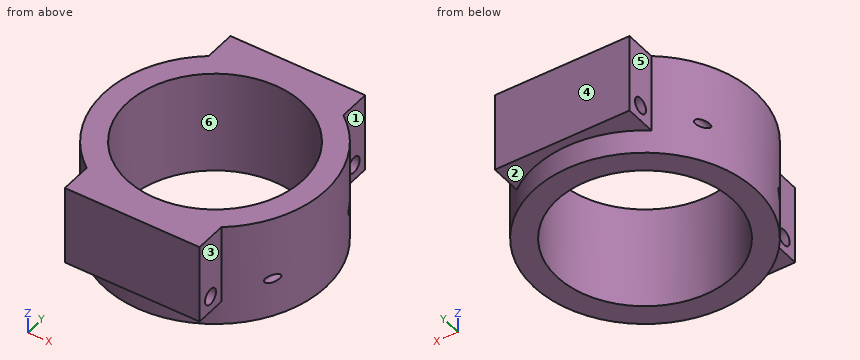
```python
from build123d import *

# Parameters (mm, degrees)
SKETCH_R           = 14
PAD_DEPTH          = 13
SKETCH001_R        = 11.1
POCKET_DEPTH       = 13.001
SKETCH002_W        = 17
SKETCH002_H        = 4
PAD001_DEPTH       = 10
POLARPATTERN_COUNT = 2
SKETCH003_R        = 0.5
POCKET001_DEPTH    = 111.473218
SKETCH004_R        = 1
POCKET002_DEPTH    = 110.373218


with BuildPart() as part:
    # Sketch → Pad (new body)
    with BuildSketch(Plane.XY):
        Circle(SKETCH_R)
    extrude(amount=PAD_DEPTH)

    # Sketch001 → Pocket (cut, through all)
    with BuildSketch(Plane.XY.offset(13)):
        Circle(SKETCH001_R)
    extrude(amount=-POCKET_DEPTH, mode=Mode.SUBTRACT)

    # Sketch002 → Pad001 (new body)
    with BuildSketch(Plane.XY.offset(13)):
        with Locations((0, 13.1)):
            Rectangle(SKETCH002_W, SKETCH002_H)
    pad001 = extrude(amount=-PAD001_DEPTH)

    # PolarPattern: Pad001 ×2 about axis
    polarpattern_axis = Axis((0, 0, 13), (0, 0, 1))
    for i in range(1, POLARPATTERN_COUNT):
        add(pad001.rotate(polarpattern_axis, i * 360 / POLARPATTERN_COUNT))

    # Sketch003 → Pocket001 (cut, through all)
    with BuildSketch(Plane.XZ.offset(10)):
        with Locations((12.1, 5)):
            Circle(SKETCH003_R)
    pocket001 = extrude(amount=-POCKET001_DEPTH, mode=Mode.SUBTRACT)

    # Mirrored: Pocket001 across Sketch003 V_Axis
    add(pocket001.mirror(Plane(origin=(0, -10, 0), x_dir=(0, -1, 0), z_dir=(1, 0, 0))), mode=Mode.SUBTRACT)

    # Sketch004 → Pocket002 (cut, through all)
    with BuildSketch(Plane(origin=(-10, 0, 0), x_dir=(0, -1, 0), z_dir=(-1, 0, 0))):
        with Locations((13.1, 5)):
            Circle(SKETCH004_R)
    pocket002 = extrude(amount=-POCKET002_DEPTH, mode=Mode.SUBTRACT)

    # Mirrored001: Pocket002 across Sketch004 V_Axis
    add(pocket002.mirror(Plane(origin=(-10, 0, 0), x_dir=(-1, 0, 0), z_dir=(0, -1, 0))), mode=Mode.SUBTRACT)


solid = part.part
```
The model under review builds one solid part; all positions refer to its coordinate system, in mm. Face numbers are marked on the shaded views. A direction names the side the tool comes from. Give positions to 0.01 mm unless a question says otherwise; leave off trailing zeros. Write each loop counter-clockwise with the first axis right and the second up, starting at its lowest first coordinate (ties: lowest second). Pieces come first, ordered by that corner, then holes. Notation, with made-up numbers: (2, 13) -> (33, 13) arc R3 cw to (33, 18) -> close; hole circle Ø10 at (-32.75, 58.5). An arc over 180 degrees is marked (long way). Put each result on its own line as item: value.
(1) To check wall thickness, follow probe 1 along X at (y, z) = (3.25, 5); probe 2 along X at (y, z) = (0, 5.25); probe 3 along Y at (x, z) = (0, 10.25). State the ranges of each line that lie inside material, in increasing order. Write a range as from..to.
Results are:
probe 1: -13.62..-12.6, -11.6..-10.61, 10.61..11.6, 12.6..13.62
probe 2: -14..-12.53, -11.67..-11.1, 11.1..11.67, 12.53..14
probe 3: -15.1..-11.1, 11.1..15.1
(2) The part is to be moulded in two halves that separate along Y. For the marked faces 4, 5 and 6, say which applies: pulls with the +Y half, pulls with the -Y half, needs draft (parallel to the pull), parting line crosses it, or undercut.
Results are:
face 4: pulls with the +Y half
face 5: needs draft
face 6: undercut
(3) We need section A-A, the plane y = 0. Give the boundary of the cut face in (x, z).
Results are:
outline: (-14, 0) -> (-11.1, 0) -> (-11.1, 13) -> (-14, 13) -> close; (11.1, 0) -> (14, 0) -> (14, 13) -> (11.1, 13) -> close; hole circle Ø1 at (-12.1, 5); hole circle Ø1 at (12.1, 5)
(4) We need section B-B, the plane z = 5. Give the boundary of the cut face in (x, y), and give its area (3 significant figures).
Results are:
outline: (-12.6, -6.1) -> (-12.6, 6.1) arc R14 ccw to start; (-11.6, -7.84) arc R14 ccw to (-8.5, -11.12) -> (-8.5, -12.1) -> (8.5, -12.1) -> (8.5, -11.12) arc R14 ccw to (11.6, -7.84) -> (11.6, 7.84) arc R14 ccw to (8.5, 11.12) -> (8.5, 12.1) -> (-8.5, 12.1) -> (-8.5, 11.12) arc R14 ccw to (-11.6, 7.84) -> close; (-8.5, -15.1) -> (8.5, -15.1) -> (8.5, -14.1) -> (-8.5, -14.1) -> close; (-8.5, 14.1) -> (8.5, 14.1) -> (8.5, 15.1) -> (-8.5, 15.1) -> close; (12.6, -6.1) arc R14 ccw to (12.6, 6.1) -> close; hole circle Ø22.2 at (0, 0)
area: 201 mm²
(5) For pin 1 Ø4.5 at (y, z) = (13.5, 9) entering from +X; pin 2 Ø2 at (y, z) = (5.5, 6.5) entering from +X; pin 3 Ø1.2 at (y, z) = (14, 8) entering from -X, all flat-tipped, find the tip position at first contact; note any pin that passes through.
Results are:
pin 1: x = 8.5
pin 2: x = 13.26
pin 3: x = -8.5
(6) We need section D-D, the plane z = 11.5. Give the boundary of the cut face in (x, y), and give its area (3 significant figures).
Results are:
outline: (-8.5, -15.1) -> (8.5, -15.1) -> (8.5, -11.12) arc R14 ccw to (8.5, 11.12) -> (8.5, 15.1) -> (-8.5, 15.1) -> (-8.5, 11.12) arc R14 ccw to (-8.5, -11.12) -> close; hole circle Ø22.2 at (0, 0)
area: 297 mm²
(7) We need section C-C, the plane x = -1.25. Give the boundary of the cut face in (y, z), and give its area (3 significant figures).
Results are:
outline: (-15.1, 3) -> (-13.94, 3) -> (-13.94, 0) -> (-11.03, 0) -> (-11.03, 13) -> (-15.1, 13) -> close; (11.03, 0) -> (13.94, 0) -> (13.94, 3) -> (15.1, 3) -> (15.1, 13) -> (11.03, 13) -> close; hole circle Ø2 at (-13.1, 5); hole circle Ø2 at (13.1, 5)
area: 92.6 mm²
(8) Tool access review of the marked faces 1, 2 and 3: name each direction out of +Z, -Z, +X, -X, +Y, -Y from which nothing blocks a thin tool from reaching the whole face with its end or side.
Results are:
face 1: +Z, -Z, +X, +Y
face 2: -Z, +Y
face 3: +Z, -Z, +X, -Y
